Could you check a few things on this model? Use its own coordinates, in mm. A direction names the side the tool comes from. Give positions to 0.01 mm unless a question says otherwise; leave off trailing zeros. Write each loop counter-clockwise with the first axis right and the second up, starting at its lowest first coordinate (ties: lowest second). Pieces come first, ordered by that corner, then holes. Notation, with made-up numbers: M 12,-4 L 41,-4 A13 cw 41,3 Z; hole C -39.5,52 d3. An arc over 180 degrees is marked long. One line per item, written item: value.
```python
from build123d import *

# Parameters (mm, degrees)
BOSS_EXTRUDE1_DEPTH = 14.5
FILLET2_R           = 14.5


with BuildPart() as part:
    # Sketch1 → Boss-Extrude1 (new, symmetric)
    with BuildSketch(Plane.YZ):
        Polygon((0, 0), (0, 62), (30, 62), (30, 15), (65, 15), (65, 0), align=None)
    extrude(amount=BOSS_EXTRUDE1_DEPTH, both=True)

    # Fillet2
    fillet2_edges = [part.edges().sort_by_distance(p)[0] for p in [
        (-14.5, 65, 7.5),
        (14.5, 65, 7.5),
    ]]
    fillet(fillet2_edges, radius=FILLET2_R - 0.0001)  # a hair under: the kernel refuses the full size


solid = part.part
```
1) Please list where these lines run through material, in increasing order: L1, parallel to Y at x = -10, z = 53.5; L2, parallel to Z at x = -8.75, y = 47.5; L3, parallel to Y at x = 1.5, z = 6.5. Write a range as from..to.
Outcome:
L1: y = 0..30
L2: z = 0..15
L3: y = 0..64.92
2) If we section it at B-B, the plane x = -7.25: Write out the boundary of the cut face in (y, z).
Outcome:
outline: M 0,0 L 63.06,0 L 63.06,15 L 30,15 L 30,62 L 0,62 Z
3) I'm going to push a flat-ended pin straight in: pin 1 (14.5 mm diameter, centred on x = -4.5, z = 43.5, fed in from +Y). Where does the tip first touch, or does it pass through?
Outcome:
pin 1: stops at y = 30
4) On a 3-axis mill with a long thin cutter (end or side, diameter ignored), from which of +Z, -Z, +X, -X, +Y, -Y can I reach the whole of each face in a straight line? I mean faces 1 (the face through (10, 61, 7)), 2 (the face through (0, 47, 15)). Say none if no direction works.
Outcome:
face 1: +Z, -Z, +X, +Y
face 2: +Z, +X, -X, +Y
5) If we section it at C-C, the plane y = 39: Write out the boundary of the cut face in (x, z).
Outcome:
outline: M -14.5,0 L 14.5,0 L 14.5,15 L -14.5,15 Z
6) If we section it at D-D, the plane x = 1.25: Write out the boundary of the cut face in (y, z), then the cut area to 3 significant figures.
Outcome:
outline: M 0,0 L 64.95,0 L 64.95,15 L 30,15 L 30,62 L 0,62 Z
area: 2,380 mm^2
7) If we section it at A-A, the plane z = 29: Write out the boundary of the cut face in (x, y).
Outcome:
outline: M -14.5,0 L 14.5,0 L 14.5,30 L -14.5,30 Z
